Here's how the part is built. I have some questions about the finished solid (model axes, mm). A direction names the side the tool comes from. Give positions to 0.01 mm unless a question says otherwise; leave off trailing zeros. Write each loop counter-clockwise with the first axis right and the second up, starting at its lowest first coordinate (ties: lowest second). Pieces come first, ordered by that corner, then holes. Notation, with made-up numbers: (-17.75, 45.5) - (7.25, 45.5) arc R6 ccw to (7.25, 53.5) - close; hole circle Ø3 at (-33, -13.75). An arc over 180 degrees is marked (long way). One line per item, written item: value. Start each with the question number.
1) Imagine slicing it at C-C on z = 1.55. Write out the boundary of the cut face in (x, y), plus the area to 3 significant figures.
2) Please list where these lines run through material, in increasing order: L1, parallel to Y at x = 0, z = 4.75; L2, parallel to Y at x = 0, z = 0.15; L3, parallel to Z at x = 5.5, y = -2. Write a range as [from, to].
3) I'm going to push flat-ended pins straight in: P1, Ø1, axis at x = 2.5, z = 4, coming from the +Y side; P2, Ø2, axis at x = 3, z = 3.5, coming from the -Y side. Where does each tip first touch, or does it pass through?
4) We'd pull the mould along Y, two halves only. Please class faces 4 (the cylindrical face through (0.867, -3.905, 2.366)), 5 (the cylindrical face through (-5.75, 5.27, 4.41)), 6 (the flat face through (-6, 4, 4)): +Y half, -Y half, draft (parallel to the pull), parting line (faces both ways), or undercut.
5) On a 3-axis mill with a long thin cutter (end or side, diameter ignored), from which of +Z, -Z, +X, -X, +Y, -Y can I reach the whole of each face in a straight line? I mean faces 1 (the flat face through (-3, -4, 0.2)), 2 (the flat face through (-2, 4, 4.8)), 3 (the flat face through (1, 5, 4.6)). Say none if no direction works.
from build123d import *

# Parameters (mm, degrees)
SKETCH_1_R          = 7
EXTRUDE_1_DEPTH     = 4.8
SKETCH_2_R          = 7.8
EXTRUDE_2_DEPTH     = 0.8
SKETCH_3_R          = 4
CUT_EXTRUDE_1_DEPTH = 5.8
SKETCH_4_R          = 6.2
SKETCH_4_R_2        = 4.8
CUT_EXTRUDE_2_DEPTH = 0.2
SKETCH_5_R          = 6.4
SKETCH_5_R_2        = 4.8
CUT_EXTRUDE_3_DEPTH = 0.2
FILLET_1_R          = 0.1


with BuildPart() as part:
    # 草圖1 → 填料-伸長1 (new body)
    with BuildSketch(Plane.XY):
        Circle(SKETCH_1_R)
    extrude(amount=EXTRUDE_1_DEPTH)

    # 草圖2 → 填料-伸長2 (add)
    with BuildSketch(Plane.XY.offset(4.8)):
        Circle(SKETCH_2_R)
    extrude(amount=-EXTRUDE_2_DEPTH)

    # 草圖3 → 除料-伸長1 (cut, through all)
    with BuildSketch(Plane(origin=(0, 0, 0), x_dir=(-1, 0, 0), z_dir=(0, 0, -1))):
        Circle(SKETCH_3_R)
    extrude(amount=-CUT_EXTRUDE_1_DEPTH, mode=Mode.SUBTRACT)

    # 草圖4 → 除料-伸長2 (cut)
    with BuildSketch(Plane(origin=(0, 0, 0), x_dir=(-1, 0, 0), z_dir=(0, 0, -1))):
        Circle(SKETCH_4_R)
        Circle(SKETCH_4_R_2, mode=Mode.SUBTRACT)
    extrude(amount=-CUT_EXTRUDE_2_DEPTH, mode=Mode.SUBTRACT)

    # 草圖5 → 除料-伸長3 (cut)
    with BuildSketch(Plane.XY.offset(4.8)):
        Circle(SKETCH_5_R)
        Circle(SKETCH_5_R_2, mode=Mode.SUBTRACT)
    extrude(amount=-CUT_EXTRUDE_3_DEPTH, mode=Mode.SUBTRACT)

    # 圓角1
    fillet_1_edges = [part.edges().sort_by_distance(p)[0] for p in [
        (-7, 0, 0),
    ]]
    fillet(fillet_1_edges, radius=FILLET_1_R)


solid = part.part
Numbers:
1. outline: circle Ø14 at (0, 0); hole circle Ø8 at (0, 0)
1. area: 104 mm^2
2. L1: [-7.8, -6.4], [-4.8, -4], [4, 4.8], [6.4, 7.8]
2. L2: [-7, -6.2], [-4.8, -4], [4, 4.8], [6.2, 7]
2. L3: [0.2, 4.6]
3. P1: y = 7.54
3. P2: y = -7.5
4. face 4: undercut
4. face 5: parting line
4. face 6: draft
5. face 1: -Z
5. face 2: +Z, +X, -X, +Y, -Y
5. face 3: +Z
